Read the model definition and answer for the solid it produces. Units are mm, in the model's axes. Face numbers are marked on the shaded views. Give positions to 0.01 mm unless a question says otherwise; leave off trailing zeros. Loops run counter-clockwise (first coordinate to the right, second up) from the corner with the lowest first, then second, coordinate; pieces in that order, holes last. Notation, with made-up numbers: (-40, 48.25) - (-26, 48.25) arc R25 cw to (-26, 83.25) - close; hole circle Ø2 at (-22.5, -20). An arc over 180 degrees is marked (long way). Use a Markdown table: item, result. Add a question column.
Item 1: A cutting plane is placed at C-C (x = 40). Determine the outline of the cut face in (y, z).
Item 2: Each of these flat-tipped pins is pushed along its axis until it touches: P1, Ø5.5, axis at x = 55, y = 28, coming from the -Z side; P2, Ø3, axis at x = 54, y = 4.5, coming from the +Z side; P3, Ø1, axis at x = 43.5, y = 14.5, coming from the +Z side; P4, Ø2.5, axis at x = 54.5, y = 4, coming from the -Z side. Where does it stop, or does it pass through?
Item 3: Consider probe 1 along Y at (x, z) = (54.6, 4.05); probe 2 along Y at (x, z) = (4.9, 0.65); probe 3 along Y at (x, z) = (18.5, 2.55). Determine where each line is inside the solid, lowest interval first. Write a range as [from, to].
Item 4: A cutting plane is placed at B-B (y = 13.5). Determine the outline of the cut face in (x, z).
Item 5: A cutting plane is placed at D-D (z = 3.45). Give the number of separate pieces and of enclosed holes in the cut face, plus the area to 3 significant figures.
Item 6: For a pull along Y with two mould halves and no side action, classify the marked faces 1, 2 and 3 as +Y half, -Y half, draft (parallel to the pull), parting line (faces both ways), or undercut.
Item 7: A cutting plane is placed at A-A (z = 0.8). Determine the outline of the cut face in (x, y), plus the area to 3 significant figures.
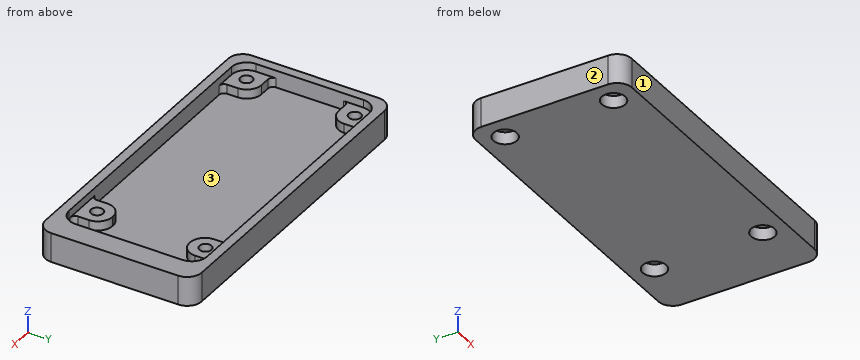
from build123d import *

# Parameters (mm, degrees)
EXTRUDE_1_DEPTH     = 6
CUT_EXTRUDE_1_DEPTH = 3.5
EXTRUDE_2_DEPTH     = 1.9
SKETCH_4_R          = 1.25
CUT_EXTRUDE_2_DEPTH = 7
SKETCH_11_R         = 2.4
CUT_EXTRUDE_3_DEPTH = 2.5
FILLET_1_R          = 1


with BuildPart() as part:
    # Эскиз1 → Бобышка-Вытянуть1 (new body)
    with BuildSketch(Plane.XY):
        with BuildLine():
            Line((3, 0), (63.8, 0))
            ThreePointArc((63.8, 0), (65.921320344, 0.878679656), (66.8, 3))
            Line((66.8, 3), (66.8, 29))
            ThreePointArc((66.8, 29), (65.921320344, 31.121320344), (63.8, 32))
            Line((63.8, 32), (3, 32))
            ThreePointArc((3, 32), (0.878679656, 31.121320344), (0, 29))
            Line((0, 29), (0, 3))
            ThreePointArc((0, 3), (0.878679656, 0.878679656), (3, 0))
        make_face()
    extrude(amount=EXTRUDE_1_DEPTH)

    # Эскиз2 → Вырез-Вытянуть1 (cut)
    with BuildSketch(Plane.XY.offset(6)):
        with BuildLine():
            Line((5, 30.1), (59, 30.1))
            ThreePointArc((59, 30.1), (61.192031022, 29.192031022), (62.1, 27))
            Line((62.1, 27), (62.1, 5))
            ThreePointArc((62.1, 5), (61.192031022, 2.807968978), (59, 1.9))
            Line((59, 1.9), (5, 1.9))
            ThreePointArc((5, 1.9), (2.807968978, 2.807968978), (1.9, 5))
            Line((1.9, 5), (1.9, 27))
            ThreePointArc((1.9, 27), (2.807968978, 29.192031022), (5, 30.1))
        make_face()
    extrude(amount=-CUT_EXTRUDE_1_DEPTH, mode=Mode.SUBTRACT)

    # Эскиз3 → Бобышка-Вытянуть2 (add)
    with BuildSketch(Plane.XY.offset(2.5)):
        with BuildLine():
            Line((4.9, 30.1), (8.1, 30.1))
            Line((8.1, 30.1), (8.1, 26.9))
            ThreePointArc((8.1, 26.9), (7.221320344, 24.778679656), (5.1, 23.9))
            Line((5.1, 23.9), (1.9, 23.9))
            Line((1.9, 23.9), (1.9, 27.1))
            ThreePointArc((1.9, 27.1), (2.778679656, 29.221320344), (4.9, 30.1))
        make_face()
        with BuildLine():
            Line((1.9, 8.1), (5.1, 8.1))
            ThreePointArc((5.1, 8.1), (7.221320344, 7.221320344), (8.1, 5.1))
            Line((8.1, 5.1), (8.1, 1.9))
            Line((8.1, 1.9), (4.9, 1.9))
            ThreePointArc((4.9, 1.9), (2.778679656, 2.778679656), (1.9, 4.9))
            Line((1.9, 4.9), (1.9, 8.1))
        make_face()
        with BuildLine():
            Line((51.5, 30.1), (57.7, 30.1))
            Line((57.7, 30.1), (57.7, 26.9))
            ThreePointArc((57.7, 26.9), (56.821320344, 24.778679656), (54.7, 23.9))
            Line((54.7, 23.9), (54.5, 23.9))
            ThreePointArc((54.5, 23.9), (52.378679656, 24.778679656), (51.5, 26.9))
            Line((51.5, 26.9), (51.5, 30.1))
        make_face()
        with BuildLine():
            Line((51.5, 1.9), (57.7, 1.9))
            Line((57.7, 1.9), (57.7, 5.1))
            ThreePointArc((57.7, 5.1), (56.821320344, 7.221320344), (54.7, 8.1))
            Line((54.7, 8.1), (54.5, 8.1))
            ThreePointArc((54.5, 8.1), (52.378679656, 7.221320344), (51.5, 5.1))
            Line((51.5, 5.1), (51.5, 1.9))
        make_face()
    extrude(amount=EXTRUDE_2_DEPTH)

    # Эскиз4 → Вырез-Вытянуть2 (cut, through all)
    with BuildSketch(Plane(origin=(0, 0, 0), x_dir=(-1, 0, 0), z_dir=(0, 0, -1))):
        with Locations((-54.6, 27.1)):
            Circle(SKETCH_4_R)
        with Locations((-4.9, 27.1)):
            Circle(SKETCH_4_R)
        with Locations((-4.9, 4.9)):
            Circle(SKETCH_4_R)
        with Locations((-54.6, 4.9)):
            Circle(SKETCH_4_R)
    extrude(amount=-CUT_EXTRUDE_2_DEPTH, mode=Mode.SUBTRACT)

    # Эскиз11 → Вырез-Вытянуть3 (cut)
    with BuildSketch(Plane(origin=(0, 0, 0), x_dir=(-1, 0, 0), z_dir=(0, 0, -1))):
        with Locations((-54.6, 27.1)):
            Circle(SKETCH_11_R)
        with Locations((-4.9, 27.1)):
            Circle(SKETCH_11_R)
        with Locations((-54.6, 4.9)):
            Circle(SKETCH_11_R)
        with Locations((-4.9, 4.9)):
            Circle(SKETCH_11_R)
    extrude(amount=-CUT_EXTRUDE_3_DEPTH, mode=Mode.SUBTRACT)

    # Скругление1
    fillet_1_edges = [part.edges().sort_by_distance(p)[0] for p in [
        (1.9, 8.1, 3.45),
        (8.1, 1.9, 3.45),
        (1.9, 23.9, 3.45),
        (8.1, 30.1, 3.45),
        (51.5, 30.1, 3.45),
        (57.7, 30.1, 3.45),
        (51.5, 1.9, 3.45),
        (57.7, 1.9, 3.45),
    ]]
    fillet(fillet_1_edges, radius=FILLET_1_R)


solid = part.part
Geometry says:
| question | item | result |
|---|---|---|
| 1 | outline | (0, 0) - (32, 0) - (32, 6) - (30.1, 6) - (30.1, 2.5) - (1.9, 2.5) - (1.9, 6) - (0, 6) - close |
| 2 | P1 | z = 0 |
| 2 | P2 | z = 4.4 |
| 2 | P3 | z = 2.5 |
| 2 | P4 | z = 2.5 |
| 3 | probe 1 | [0, 3.65], [6.15, 8.1], [23.9, 25.85], [28.35, 32] |
| 3 | probe 2 | [0, 2.5], [7.3, 24.7], [29.5, 32] |
| 3 | probe 3 | [0, 1.9], [30.1, 32] |
| 4 | outline | (0, 0) - (66.8, 0) - (66.8, 6) - (62.1, 6) - (62.1, 2.5) - (1.9, 2.5) - (1.9, 6) - (0, 6) - close |
| 5 | separate pieces | 1 |
| 5 | enclosed holes | 5 |
| 5 | area | 561 mm² |
| 6 | face 1 | -Y half |
| 6 | face 2 | draft |
| 6 | face 3 | undercut |
| 7 | outline | (0, 3) arc R3 ccw to (3, 0) - (63.8, 0) arc R3 ccw to (66.8, 3) - (66.8, 29) arc R3 ccw to (63.8, 32) - (3, 32) arc R3 ccw to (0, 29) - close; hole circle Ø4.8 at (4.9, 4.9); hole circle Ø4.8 at (4.9, 27.1); hole circle Ø4.8 at (54.6, 4.9); hole circle Ø4.8 at (54.6, 27.1) |
| 7 | area | 2,060 mm² |
